Here's how the part is built. I have some questions about the finished solid (model axes, mm). A direction names the side the tool comes from. Coordinates: 2 decimals unless noted, no trailing zeros. Loops run counter-clockwise (first coordinate to the right, second up) from the corner with the lowest first, then second, coordinate; pieces in that order, holes last. Notation, with made-up numbers: M -5,62 L 48,62 A8 ccw 48,76 Z; hole C 71,23.25 d5. An arc over 180 degrees is marked long. Use one line per item in the form item = value. Start each with the question number.
(1) Imagine slicing it at C-C, the plane x = -11. Please give me the cut outline in (y, z), and give its area (3 significant figures).
(2) Please list where these lines run through material, in increasing order: L1, parallel to Z at x = -4, y = 140.5; L2, parallel to Y at x = -1.25, z = 57; L3, parallel to Z at x = -10.75, y = -17.5.
(3) Will these pins go through, and if not, where does the flat tip stop? P1, Ø1, axis at x = -2, y = 105.5, coming from the -Z side; P2, Ø2, axis at x = -17.5, z = -156, coming from the +Y side; P3, Ø1.5, axis at x = -6, z = -341.5, coming from the -Y side.
(4) Imagine slicing it at A-A, the plane y = 191.5. Please give me the cut outline in (x, z), and give its area (3 significant figures).
(5) Imagine slicing it at B-B, the plane z = 80. Please give me the cut outline in (x, y).
(6) On a 3-axis mill with a long thin cutter (end or side, diameter ignored), from which of +Z, -Z, +X, -X, +Y, -Y can I reach the whole of each face in a straight line? I mean faces 4 (the flat face through (-9.86, 0.767, 90.125)), 5 (the flat face through (-10, 0, -204)). Say none if no direction works.
(7) Thinking about a two-plate mould opening in Z: for faces 1 (the flat face through (-9.86, 110.87, -374.67)), 2 (the cylindrical face through (-9.86, 282.25, -292.53)), 3 (the cylindrical face through (-9.86, 146.798, 50.164)), which applies, +Z half, -Z half, draft (parallel to the pull), parting line (faces both ways), or undercut?
(8) Imagine slicing it at D-D, the plane z = -159. Please give me the cut outline in (x, y).
```python
from build123d import *

# Parameters (mm, degrees)
SKETCH1_R          = 55.5
BASE_FLANGE1_DEPTH = 20
FILLET_1_0_R       = 1


# Sheet-metal steps are written as plain solids
with BuildPart() as part:
    # Sketch1 → Base-Flange1 (new body)
    with BuildSketch(Plane(origin=(0, 0, 0), x_dir=(0, 0, -1), z_dir=(1, 0, 0))):
        with BuildLine():
            Line((0, -41), (0, -12.5))
            ThreePointArc((0, -12.5), (3.661165235, -3.661165235), (12.5, 0))
            Line((12.5, 0), (402, 0))
            Line((402, 0), (346.87955959, 223.617766639))
            ThreePointArc((346.87955959, 223.617766639), (291.405611492, 282.611111197), (212.20304892, 265.743162247))
            ThreePointArc((212.20304892, 265.743162247), (81.106216912, 192.940833045), (-68.425866876, 181.684083165))
            ThreePointArc((-68.425866876, 181.684083165), (-155.341011221, 133.615205312), (-133.058215758, 36.825038658))
            Line((-133.058215758, 36.825038658), (-45.972209781, -36.315142143))
            ThreePointArc((-45.972209781, -36.315142143), (-39.95421417, -39.792323471), (-33.109612021, -41))
            Line((-33.109612021, -41), (0, -41))
        make_face()
        with Locations((-80, 100)):
            Circle(SKETCH1_R, mode=Mode.SUBTRACT)
        with Locations((266.777160234, 203.873004866)):
            Circle(SKETCH1_R, mode=Mode.SUBTRACT)
    extrude(amount=-BASE_FLANGE1_DEPTH)

    # Fillet-1.0
    fillet_1_0_edges = [part.edges().sort_by_distance(p)[0] for p in [
        (-10, 0, -402),
        (-10, -41, 0),
    ]]
    fillet(fillet_1_0_edges, radius=FILLET_1_0_R)


solid = part.part
```
Answer:
q1.outline = M -41,1 A1 ccw -40,0 L -12.5,0 A12.5 cw 0,-12.5 L 0,-400.72 A1 ccw 1.24,-401.69 L 223.62,-346.88 A82.5 ccw 265.74,-212.2 A350 cw 181.68,68.43 A82.5 ccw 36.83,133.06 L -36.32,45.97 A20 ccw -41,33.11 Z; hole C 100,80 d111; hole C 203.87,-266.78 d111
q1.area = 96,100 mm²
q2.L1 = -367.37 to 42.05, 117.95 to 151.87
q2.L2 = -27.05 to 49.49, 150.51 to 180.26
q2.L3 = 0 to 68.37
q3.P1 = -376.12
q3.P2 = 225.88
q3.P3 = 0
q4.outline = M -20,-354.8 L 0,-354.8 L 0,-320.88 L -20,-320.88 Z; M -20,-212.67 L 0,-212.67 L 0,-76.16 L -20,-76.16 Z
q4.area = 3,410 mm²
q5.outline = M -20,-7.74 L 0,-7.74 L 0,44.5 L -20,44.5 Z; M -20,155.5 L 0,155.5 L 0,182.5 L -20,182.5 Z
q6.face_4 = +Z, +X, -X, -Y
q6.face_5 = -Z, +X, -X, -Y
q7.face_1 = -Z half
q7.face_2 = parting line
q7.face_3 = undercut
q8.outline = M -20,0 L 0,0 L 0,227.06 L -20,227.06 Z
